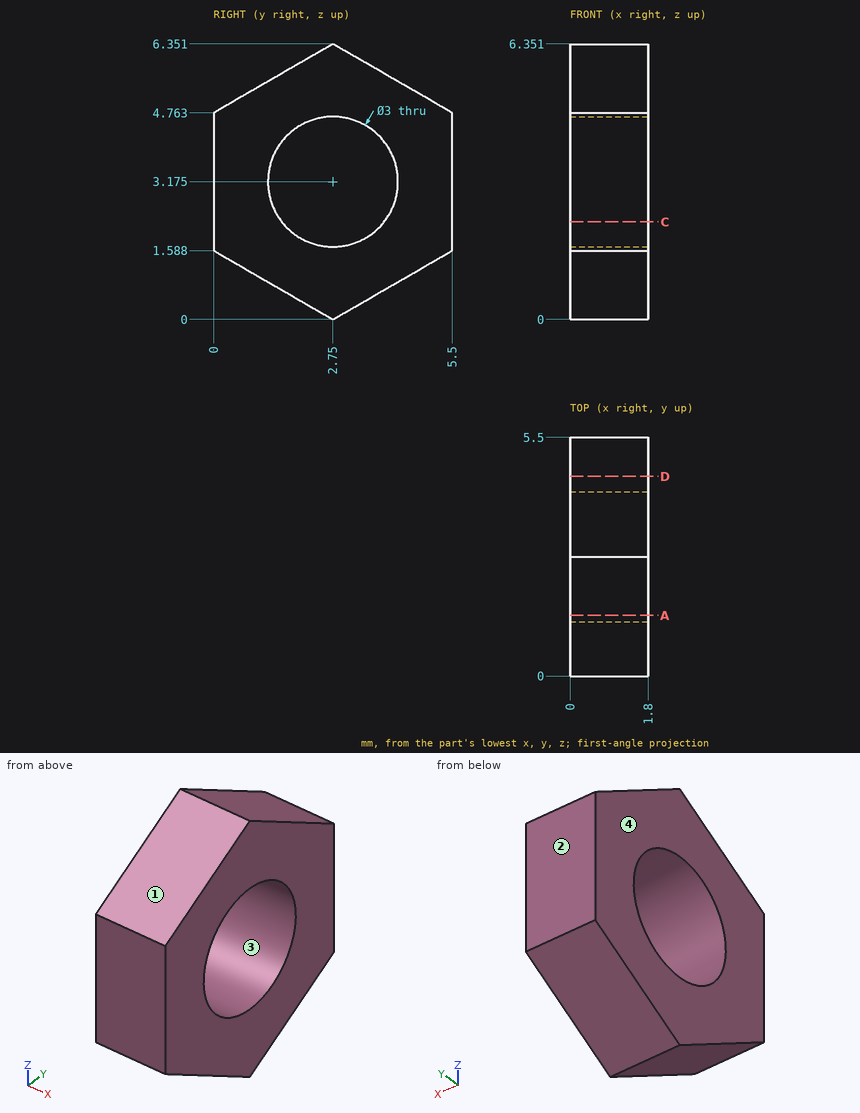
Geometry check sheet. Reference: drawing and pictorial views, mm from the part's lowest x, y, z. Give positions to 0.01 mm unless a question says otherwise; leave off trailing zeros. Write each loop counter-clockwise with the first axis right and the second up, starting at its lowest first coordinate (ties: lowest second). Pieces come first, ordered by that corner, then holes. Notation, with made-up numbers: M 19,15.25 L 50,15.25 A22 cw 50,37.25 Z; hole C -37.75,-12 d3. An arc over 180 degrees is marked long. Put each result on its own line as item: value. Start each with the question number.
1. Section check A-A (y = 1.4). Record the cut outline in (x, z).
2. Go/stop test with a flat-tipped pin: pin 1 Ø1 at (y, z) = (2.5, 4.5) entering from -X. Record where the tip stops, or that it passes through.
3. Section check D-D (y = 4.6). Record the cut outline in (x, z).
4. Scan lines: line 1 along Y through (x, z) = (0.5, 4.25) (1 decimal); line 2 along Y through (x, z) = (0.15, 2.75); line 3 along Y through (x, z) = (0.95, 5.25) (1 decimal). Record each from-to range of solid material in increasing order. Write a range as [from, to].
5. Draft check along Y on the marked faces 1, 2, 3 and 4. Enter one of: +Y half, -Y half, draft (parallel to the pull), parting line (faces both ways), or undercut.
6. Section check C-C (z = 2.25). Record the cut outline in (x, y).
Answer list:
1. outline: M 0,0.78 L 1.8,0.78 L 1.8,2.52 L 0,2.52 Z; M 0,3.83 L 1.8,3.83 L 1.8,5.57 L 0,5.57 Z
2. pin 1: x = 0
3. outline: M 0,1.07 L 1.8,1.07 L 1.8,5.28 L 0,5.28 Z
4. line 1: [0, 1.7], [3.8, 5.5]
4. line 2: [0, 1.31], [4.19, 5.5]
4. line 3: [0.8, 4.7]
5. face 1: -Y half
5. face 2: +Y half
5. face 3: undercut
5. face 4: draft
6. outline: M 0,0 L 1.8,0 L 1.8,1.57 L 0,1.57 Z; M 0,3.93 L 1.8,3.93 L 1.8,5.5 L 0,5.5 Z
